The drawing under review shows one solid part. Ordinate dimensions are in mm from its lowest x, y, z. Coordinates: 2 decimals unless noted, no trailing zeros. Loops run counter-clockwise (first coordinate to the right, second up) from the corner with the lowest first, then second, coordinate; pieces in that order, holes last. Notation, with made-up numbers: M 73,46 L 111,46 A16 cw 111,74 Z; hole C -37.5,-13.75 d1. An arc over 180 degrees is marked long. Put each result on its own line as item: value.
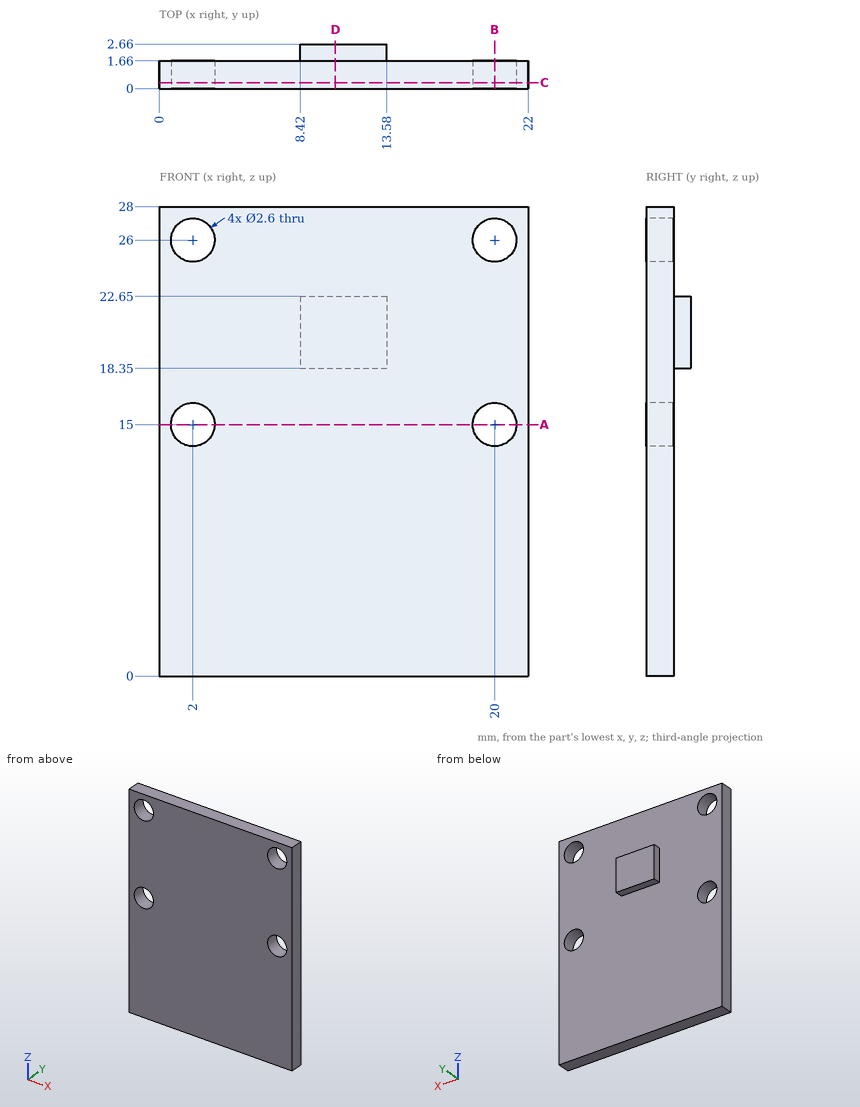
(1) Add section C-C (y = 0.35). Write out the cut boundary in (x, z), plus the area to 3 significant figures.
Determined:
outline: M 0,0 L 22,0 L 22,28 L 0,28 Z; hole C 2,15 d2.6; hole C 2,26 d2.6; hole C 20,15 d2.6; hole C 20,26 d2.6
area: 595 mm^2
(2) Wall thickness on line 1 along Z through (x, y) = (2, 1.1); line 2 along X through (y, z) = (1.15, 15); line 3 along X through (y, z) = (0.85, 25.5): over which ranges is each line inside the solid? List them lowest first. Write a range as [from, to].
Determined:
line 1: z = [0, 13.7], [16.3, 24.7], [27.3, 28]
line 2: x = [0, 0.7], [3.3, 18.7], [21.3, 22]
line 3: x = [0, 0.8], [3.2, 18.8], [21.2, 22]
(3) Add section B-B (x = 20). Write out the cut boundary in (y, z), plus the area to 3 significant figures.
Determined:
outline: M 0,0 L 1.66,0 L 1.66,13.7 L 0,13.7 Z; M 0,16.3 L 1.66,16.3 L 1.66,24.7 L 0,24.7 Z; M 0,27.3 L 1.66,27.3 L 1.66,28 L 0,28 Z
area: 37.8 mm^2
(4) Add section D-D (x = 10.5). Write out the cut boundary in (y, z).
Determined:
outline: M 0,0 L 1.66,0 L 1.66,18.35 L 2.66,18.35 L 2.66,22.65 L 1.66,22.65 L 1.66,28 L 0,28 Z
(5) For pin 1 (11 mm diameter, centred on x = 8, z = 8.5, fed in from +Y); pin 2 (1.1 mm diameter, centred on x = 10.5, y = 2.5, fed in from +Z); pin 3 (1 mm diameter, centred on x = 10, y = 0.5, fed in from -Z); pin 4 (0.8 mm diameter, centred on x = 12, y = 2.5, fed in from -Z), all flat-tipped, find the tip position at first contact; note any pin that passes through.
Determined:
pin 1: stops at y = 1.66
pin 2: stops at z = 22.65
pin 3: stops at z = 0
pin 4: stops at z = 18.35
(6) Add section A-A (z = 15). Write out the cut boundary in (x, y), plus the area to 3 significant figures.
Determined:
outline: M 0,0 L 0.7,0 L 0.7,1.66 L 0,1.66 Z; M 3.3,0 L 18.7,0 L 18.7,1.66 L 3.3,1.66 Z; M 21.3,0 L 22,0 L 22,1.66 L 21.3,1.66 Z
area: 27.9 mm^2
